```python
from build123d import *

# Parameters (mm, degrees)
SKETCH1_W            = 127
SKETCH1_H            = 76.2
PLATE_DEPTH          = 6.35
SKETCH2_R            = 3.175
CUT_EXTRUDE1_DEPTH   = 75.324844433
LPATTERN1_COUNT      = 2
LPATTERN1_PITCH      = 101.6
LPATTERN1_COUNT_DIR2 = 2
LPATTERN1_PITCH_DIR2 = 50.8
SKETCH4_R            = 12.7
CUT_EXTRUDE2_DEPTH   = 75.324844433
FILLET1_R            = 6.35


with BuildPart() as part:
    # Sketch1 → Plate (new body)
    with BuildSketch(Plane(origin=(0, 0, 0), x_dir=(1, 0, 0), z_dir=(0, 1, 0))):
        Rectangle(SKETCH1_W, SKETCH1_H)
    extrude(amount=PLATE_DEPTH)

    # Sketch2 → Cut-Extrude1 (cut, through all)
    with BuildSketch(Plane(origin=(0, 6.35, 0), x_dir=(1, 0, 0), z_dir=(0, 1, 0))):
        with Locations(Location((50.8, 25.4, 0), (0, 0, 270))):
            Circle(SKETCH2_R)
    cut_extrude1 = extrude(amount=-CUT_EXTRUDE1_DEPTH, mode=Mode.SUBTRACT)

    # LPattern1: Cut-Extrude1 2 × 2
    with Locations(*[(-i * LPATTERN1_PITCH, 0, j * LPATTERN1_PITCH_DIR2) for i in range(LPATTERN1_COUNT) for j in range(LPATTERN1_COUNT_DIR2) if (i, j) != (0, 0)]):
        add(cut_extrude1, mode=Mode.SUBTRACT)

    # Sketch4 → Cut-Extrude2 (cut, through all)
    with BuildSketch(Plane(origin=(0, 6.35, 0), x_dir=(1, 0, 0), z_dir=(0, 1, 0))):
        with Locations(Location((0, 0, 0), (0, 0, 270))):
            Circle(SKETCH4_R)
    extrude(amount=-CUT_EXTRUDE2_DEPTH, mode=Mode.SUBTRACT)

    # Fillet1
    fillet1_edges = [part.edges().sort_by_distance(p)[0] for p in [
        (-63.5, 3.175, -38.1),
        (63.5, 3.175, -38.1),
        (63.5, 3.175, 38.1),
        (-63.5, 3.175, 38.1),
    ]]
    fillet(fillet1_edges, radius=FILLET1_R)


solid = part.part
```
Input: part model. Units: mm. Frame: model coordinates. Round coordinates to 2 decimals unless told otherwise and drop trailing zeros. Write each loop counter-clockwise with the first axis right and the second up, starting at its lowest first coordinate (ties: lowest second). Pieces come first, ordered by that corner, then holes. Notation, with made-up numbers: M 8,52.5 L 31,52.5 A32 cw 31,88.5 Z; hole C 69.25,-13.75 d8. An arc over 180 degrees is marked long. Write each question's results on one line, items separated by ' | '.
Q1. Section query B-B (z = 25.4). Return loops of the section in (x, y) (3 decimals), and give its area (3 significant figures).
Results:
outline: M -63.5,0 L -53.975,0 L -53.975,6.35 L -63.5,6.35 Z; M -47.625,0 L 47.625,0 L 47.625,6.35 L -47.625,6.35 Z; M 53.975,0 L 63.5,0 L 63.5,6.35 L 53.975,6.35 Z | area: 726 mm^2
Q2. Section query C-C (y = 4.5). Return loops of the section in (x, z) (3 decimals).
Results:
outline: M -63.5,-31.75 A6.35 ccw -57.15,-38.1 L 57.15,-38.1 A6.35 ccw 63.5,-31.75 L 63.5,31.75 A6.35 ccw 57.15,38.1 L -57.15,38.1 A6.35 ccw -63.5,31.75 Z; hole C -50.8,-25.4 d6.35; hole C -50.8,25.4 d6.35; hole C 0,0 d25.4; hole C 50.8,-25.4 d6.35; hole C 50.8,25.4 d6.35
Q3. Section query D-D (z = 0). Return loops of the section in (x, y), and give its area (3 significant figures).
Results:
outline: M -63.5,0 L -12.7,0 L -12.7,6.35 L -63.5,6.35 Z; M 12.7,0 L 63.5,0 L 63.5,6.35 L 12.7,6.35 Z | area: 645 mm^2
Q4. Line query: line 1 along X through (y, z) = (3.5, -25.4) (3 decimals); line 2 along X through (y, z) = (4.75, 27); line 3 along Z through (x, y) = (51, 0.5). Output: solid intervals per line, ascending.
Results:
line 1: x = -63.5 to -53.975, -47.625 to 47.625, 53.975 to 63.5 | line 2: x = -63.5 to -53.54, -48.06 to 48.06, 53.54 to 63.5 | line 3: z = -38.1 to -28.57, -22.23 to 22.23, 28.57 to 38.1
Q5. Pin query (flat end, axial travel): P1, Ø4, axis at x = 50.8, z = 25.4, coming from the -Y side; P2, Ø8.5, axis at x = -50.8, z = -25.4, coming from the +Y side. Return the tip coordinate at first contact, or that it passes through.
Results:
P1: passes through | P2: stops at y = 6.35
Q6. Draft query along Z for faces 1 (the face through (-1, 3, 38.1)), 2 (the face through (-7.7, 3.2, -10.1)), 3 (the face through (13, 0, -1)). Return one class per face: released by +Z, released by -Z, zero draft, split by the parting line, or undercut.
Results:
face 1: released by +Z | face 2: undercut | face 3: zero draft
Q7. Section query A-A (x = 0). Return loops of the section in (y, z), and give its area (3 significant figures).
Results:
outline: M 0,-38.1 L 6.35,-38.1 L 6.35,-12.7 L 0,-12.7 Z; M 0,12.7 L 6.35,12.7 L 6.35,38.1 L 0,38.1 Z | area: 323 mm^2
